Can you work these out from the model? Positions are in its coordinate system, mm. Face numbers are marked on the shaded views. A direction names the side the tool comes from. Coordinates: 2 decimals unless noted, no trailing zeros. Order: outer loops, then holes, each group sorted by start corner. A loop starts at its lowest first (then second) coordinate and runs counter-clockwise, first axis right, second up. Notation, with made-up numbers: (72, 2.5) - (85, 2.5) arc R11 cw to (85, 12.5) - close; hole circle Ø2 at (88, 40.25). An arc over 180 degrees is marked (long way). Use a Markdown table: item, result. Add a question column.
(1) I want a section at A-A (z = 13). List the corners of the cut face in (x, y) for me, and give its area (3 significant figures).
(2) On a 3-axis mill with a long thin cutter (end or side, diameter ignored), from which of +Z, -Z, +X, -X, +Y, -Y can I reach the whole of each face in a straight line? I mean the marked faces 1 and 2. Say none if no direction works.
(3) For pin 1 Ø4 at (x, z) = (-3, 12) entering from -Y; pin 2 Ø3 at (x, z) = (-5, 28) entering from -Y; pin 3 Ø3 at (y, z) = (-5, 25.5) entering from +X, each with a flat end and sliding along its axis, tell me the tip position at first contact or that it passes through.
(4) If I drill on L1, parallel to Y at x = -1, z = 6.5; L2, parallel to X at y = 2, z = 6; L3, parallel to X at y = -11.75, z = 14, over which ranges is the centre line in solid material (lowest first)? Write a range as [from, to].
```python
from build123d import *

# Parameters (mm, degrees)
SKETCH1_R           = 13.5
BOSS_EXTRUDE1_DEPTH = 32
FILLET1_R           = 2
SKETCH2_R           = 14.634398313
SKETCH2_R_2         = 12
CUT_EXTRUDE1_DEPTH  = 3
FILLET2_R           = 2


with BuildPart() as part:
    # Sketch1 → Boss-Extrude1 (new body)
    with BuildSketch(Plane.XY):
        Circle(SKETCH1_R)
    extrude(amount=BOSS_EXTRUDE1_DEPTH)

    # Fillet1
    fillet1_edges = [part.edges().sort_by_distance(p)[0] for p in [
        (-13.5, 0, 32),
    ]]
    fillet(fillet1_edges, radius=FILLET1_R)

    # Sketch2 → Cut-Extrude1 (cut)
    with BuildSketch(Plane(origin=(0, 0, 0), x_dir=(-1, 0, 0), z_dir=(0, 0, -1))):
        Circle(SKETCH2_R)
        Circle(SKETCH2_R_2, mode=Mode.SUBTRACT)
    extrude(amount=-CUT_EXTRUDE1_DEPTH, mode=Mode.SUBTRACT)

    # Fillet2
    # the kernel refuses this fillet: 2 mm, written as the material it takes off along each edge
    with BuildSketch(Plane(origin=(0, 0, 3), x_dir=(1, 0, 0), z_dir=(0, 1, 0))) as fillet2_piece_1:
        with BuildLine():
            CenterArc((11.5, -1.936491673), FILLET2_R, 0, 75.522487814)
            Line((12, 0), (12.01, 0.038729833))
            ThreePointArc((12.01, 0.038729833), (12.75, 0.04), (13.5, 0.04))
            Line((13.5, 0.04), (13.54, 0))
            Line((13.54, 0), (13.54, -1.936491673))
            Line((13.54, -1.936491673), (13.5, -1.936491673))
        make_face()
    revolve(axis=Axis((0, 0, 3), (0, 0, -1)), mode=Mode.SUBTRACT)


solid = part.part
```
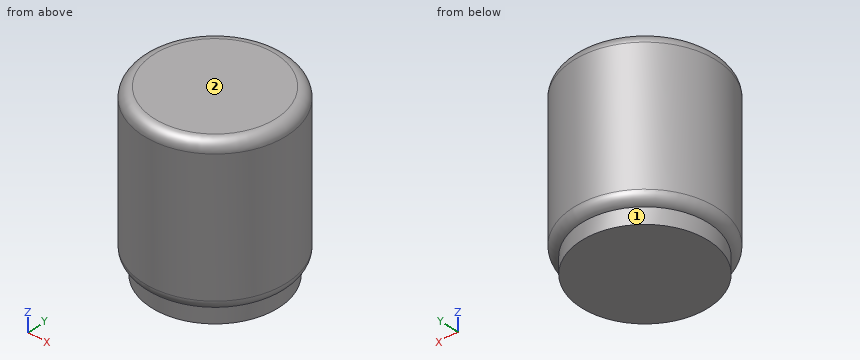
Answers follow:
| question | item | result |
|---|---|---|
| 1 | outline | circle Ø27 at (0, 0) |
| 1 | area | 573 mm² |
| 2 | face 1 | -Z |
| 2 | face 2 | +Z, +X, -X, +Y, -Y |
| 3 | pin 1 | stops at y = -13.46 |
| 3 | pin 2 | stops at y = -13.04 |
| 3 | pin 3 | stops at x = 13.04 |
| 4 | L1 | y = [-13.46, 13.46] |
| 4 | L2 | x = [-13.35, 13.35] |
| 4 | L3 | x = [-6.65, 6.65] |
